Can you work these out from the model? Positions are in its coordinate system, mm. A direction names the side the tool comes from. Coordinates: 2 decimals unless noted, no trailing zeros. Loops run counter-clockwise (first coordinate to the right, second up) from the corner with the lowest first, then second, coordinate; pieces in that order, holes last. Notation, with made-up numbers: (39.5, 41) -> (94.5, 41) arc R4 cw to (94.5, 45) -> close; hole circle Ø3 at (81.5, 14.5). An arc over 180 degrees is marked (long way). Use one line per item in the form item = value. Start each with the question number.
(1) I need wall thicknesses on line 1 (Y direction, x = -87.5, z = 5); line 2 (X direction, y = 134, z = -1). Which ranges of each line are inside material? Lowest first, please. Write a range as [from, to].
(2) On a 3-axis mill with a long thin cutter (end or side, diameter ignored), from which of +Z, -Z, +X, -X, +Y, -Y can I reach the whole of each face in a straight line? I mean faces 1 (the flat face through (-19.05, 290, 0)), 2 (the flat face through (-79, 565.15, 0)), 3 (the flat face through (-86, 558.8, 0)), 4 (the flat face through (-17, 373, -19.05)). Say none if no direction works.
(3) Thinking about a two-plate mould opening in X: for faces 5 (the flat face through (-78, 603.25, 0)), 6 (the flat face through (25.4, 334, 0)), 7 (the flat face through (-13, 373, 19.05)), 8 (the flat face through (19.05, 328, 0)), which applies, released by +X, released by -X, zero draft, split by the parting line, or undercut?
(4) Imagine slicing it at A-A (y = 132.5). List the corners of the cut face in (x, z) for me.
(5) Imagine slicing it at C-C (z = 12.5). List the corners of the cut face in (x, y) for me, plus the area to 3 significant figures.
(6) Imagine slicing it at D-D (x = -11). List the corners of the cut face in (y, z) for me.
(7) Imagine slicing it at B-B (x = -48.5). List the corners of the cut face in (y, z) for me.
(8) I'm going to push flat-ended pins straight in: pin 1 (5 mm diameter, centred on x = -51, z = 6.5, fed in from -Y); pin 2 (11.5 mm diameter, centred on y = 230.5, z = -9, fed in from -X). Where does each tip first touch, or does it pass through?
```python
from build123d import *

# Parameters (mm, degrees)
F1_W     = 50.8
F1_H     = 50.8
F1_W_2   = 38.1
F1_H_2   = 38.1
F4_DEPTH = 50.801
F6_DEPTH = 609.601


with BuildPart() as f2:
    # F2: sweep along a path in F0
    with BuildLine(Plane.XY) as f2_path:
        Line((0, 0), (0, 584.2))
        Line((0, 584.2), (-177.8, 584.2))
    # F1 (on Front) → F2 (sweep)
    with BuildSketch(Plane.XZ):
        Rectangle(F1_W, F1_H)
        Rectangle(F1_W_2, F1_H_2, mode=Mode.SUBTRACT)
    sweep(path=f2_path.line, transition=Transition.RIGHT)

    # F3 (on face) → F4 (cut, through all)
    with BuildSketch(Plane.XY.offset(25.4)):
        Polygon((-25.4, 0), (25.4, 0), (25.4, 50.8), align=None)
    extrude(amount=-F4_DEPTH, mode=Mode.SUBTRACT)

    # F5 (on face) → F6 (cut, through all)
    with BuildSketch(Plane(origin=(0, 609.6, 0), x_dir=(-1, 0, 0), z_dir=(0, 1, 0))):
        Polygon((177.8, -25.4), (177.8, 25.4), (127, -25.4), align=None)
    extrude(amount=-F6_DEPTH, mode=Mode.SUBTRACT)


solid = f2.part
```
Worked out:
q1.line_1 = [558.8, 565.15], [603.25, 609.6]
q1.line_2 = [-25.4, -19.05], [19.05, 25.4]
q2.face_1 = -Y
q2.face_2 = -X
q2.face_3 = +Z, -Z, -X, -Y
q2.face_4 = none
q3.face_5 = zero draft
q3.face_6 = released by +X
q3.face_7 = undercut
q3.face_8 = undercut
q4.outline = (-25.4, -25.4) -> (25.4, -25.4) -> (25.4, 25.4) -> (-25.4, 25.4) -> close; hole (-19.05, -19.05) -> (19.05, -19.05) -> (19.05, 19.05) -> (-19.05, 19.05) -> close
q5.outline = (-164.9, 558.8) -> (-25.4, 558.8) -> (-25.4, 0) -> (-19.05, 6.35) -> (-19.05, 565.15) -> (-164.9, 565.15) -> close; (-164.9, 603.25) -> (19.05, 603.25) -> (19.05, 44.45) -> (25.4, 50.8) -> (25.4, 609.6) -> (-164.9, 609.6) -> close
q5.area = 9,190 mm2
q6.outline = (14.4, -25.4) -> (609.6, -25.4) -> (609.6, 25.4) -> (14.4, 25.4) -> (14.4, 19.05) -> (603.25, 19.05) -> (603.25, -19.05) -> (14.4, -19.05) -> close
q7.outline = (558.8, -25.4) -> (609.6, -25.4) -> (609.6, 25.4) -> (558.8, 25.4) -> close; hole (565.15, -19.05) -> (603.25, -19.05) -> (603.25, 19.05) -> (565.15, 19.05) -> close
q8.pin_1 = 558.8
q8.pin_2 = -25.4
